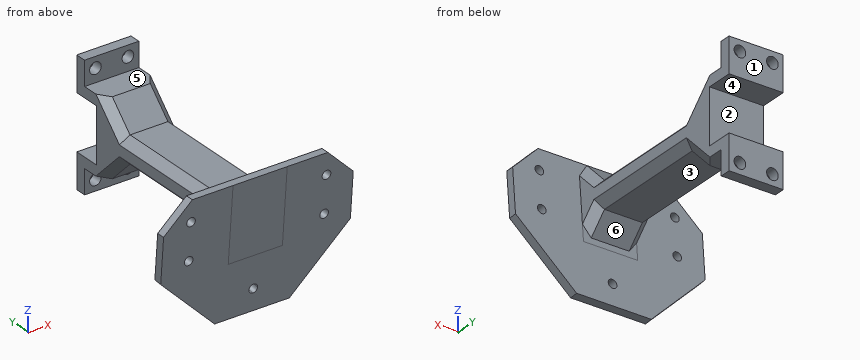
```python
from build123d import *

# Parameters (mm, degrees)
SKETCH1_W           = 20
SKETCH1_H           = 53.344530479
BOSS_EXTRUDE1_DEPTH = 28
BOSS_EXTRUDE2_START = -426.399445517
BOSS_EXTRUDE2_DEPTH = 20
BOSS_EXTRUDE3_DEPTH = 20
SKETCH4_R           = 2.15
CUT_EXTRUDE1_DEPTH  = 10
SKETCH6_R           = 1.6
BOSS_EXTRUDE5_DEPTH = 3
SKETCH7_W           = 104.374043795
SKETCH7_H           = 16.644454458
CUT_EXTRUDE2_DEPTH  = 3
CHAMFER1_SIZE       = 10
CUT_EXTRUDE3_DEPTH  = 60
CHAMFER2_SIZE       = 3


# Read off the part's stored shape, not the designer's step: Boss-Extrude2
with BuildPart() as part:
    # Sketch1 → Boss-Extrude1 (new body)
    with BuildSketch(Plane.XY):
        with Locations((-416.399445517, 267.662547877)):
            Rectangle(SKETCH1_W, SKETCH1_H)
    extrude(amount=-BOSS_EXTRUDE1_DEPTH)

    # Boss-Extrude2 outline → Boss-Extrude2 (add)
    with BuildSketch(Plane.YZ.offset(BOSS_EXTRUDE2_START)):
        Polygon((227.085747643, -28), (240.990282637, -28), (240.990282637, 0), (224.636065064, 0), align=None)
    extrude(amount=BOSS_EXTRUDE2_DEPTH)

    # Sketch3 → Boss-Extrude3 (add)
    with BuildSketch(Plane.ZY.offset(426.399445517)):
        Polygon((-28, 300.334813116), (-37, 300.334813116), (-37, 304.334813116), (-24.1, 304.334813116), (-24.1, 294.334813116), (-28, 294.334813116), align=None)
        Polygon((9, 300.334813116), (9, 304.334813116), (-3.9, 304.334813116), (-3.9, 294.334813116), (0, 294.334813116), (0, 300.334813116), align=None)
    extrude(amount=-BOSS_EXTRUDE3_DEPTH)

    # Sketch4 → Cut-Extrude1 (cut)
    with BuildSketch(Plane(origin=(0, 304.334813116, 0), x_dir=(1, 0, 0), z_dir=(0, 1, 0))):
        with Locations(Location((-422.399445517, 33, 0), (0, 0, 270))):
            Circle(SKETCH4_R)
        with Locations(Location((-410.399445517, 33, 0), (0, 0, 270))):
            Circle(SKETCH4_R)
        with Locations(Location((-410.399445517, -5, 0), (0, 0, 90))):
            Circle(SKETCH4_R)
        with Locations(Location((-422.399445517, -5, 0), (0, 0, 90))):
            Circle(SKETCH4_R)
    extrude(amount=-CUT_EXTRUDE1_DEPTH, mode=Mode.SUBTRACT)

    # Sketch6 → Boss-Extrude5 (add)
    # profile 1 of 2: a face of its own
    with BuildSketch(Plane(origin=(0, 222.929701773, 19.503821668), x_dir=(1, 0, 0), z_dir=(0, -0.9961946980917453, -0.087155742747662))):
        with BuildLine():
            Line((-426.399445517, -19.578323099), (-451.399445517, -19.578323099))
            Line((-451.399445517, -19.578323099), (-451.399445517, -46.472075114))
            Line((-451.399445517, -46.472075114), (-430.186242082, -67.68527855))
            Line((-430.186242082, -67.68527855), (-416.399445517, -67.68527855))
            Line((-416.399445517, -67.68527855), (-416.399445517, -61.28527855))
            ThreePointArc((-416.399445517, -61.28527855), (-417.999445517, -59.68527855), (-416.399445517, -58.08527855))
            Line((-416.399445517, -58.08527855), (-416.399445517, -47.68527855))
            Line((-416.399445517, -47.68527855), (-426.399445517, -47.68527855))
            Line((-426.399445517, -47.68527855), (-426.399445517, -19.578323099))
        make_face()
        with Locations(Location((-441.399445517, -41.472075114, 0), (0, 0, 270))):
            Circle(SKETCH6_R, mode=Mode.SUBTRACT)
        with Locations(Location((-441.399445517, -27.578323099, 0), (0, 0, 270))):
            Circle(SKETCH6_R, mode=Mode.SUBTRACT)
    # profile 2 of 2: a face of its own
    with BuildSketch(Plane(origin=(0, 222.929701773, 19.503821668), x_dir=(1, 0, 0), z_dir=(0, -0.9961946980917453, -0.087155742747662))):
        with BuildLine():
            Line((-416.399445517, -61.28527855), (-416.399445517, -67.68527855))
            Line((-416.399445517, -67.68527855), (-402.612648953, -67.68527855))
            Line((-402.612648953, -67.68527855), (-381.399445517, -46.472075114))
            Line((-381.399445517, -46.472075114), (-381.399445517, -19.578323099))
            Line((-381.399445517, -19.578323099), (-406.399445517, -19.578323099))
            Line((-406.399445517, -19.578323099), (-406.399445517, -47.68527855))
            Line((-406.399445517, -47.68527855), (-416.399445517, -47.68527855))
            Line((-416.399445517, -47.68527855), (-416.399445517, -58.08527855))
            ThreePointArc((-416.399445517, -58.08527855), (-415.268074667, -58.5539077), (-414.799445517, -59.68527855))
            ThreePointArc((-414.799445517, -59.68527855), (-415.268074667, -60.8166494), (-416.399445517, -61.28527855))
        make_face()
        with Locations(Location((-391.399445517, -41.472075114, 0), (0, 0, 270))):
            Circle(SKETCH6_R, mode=Mode.SUBTRACT)
        with Locations(Location((-391.399445517, -27.578323099, 0), (0, 0, 270))):
            Circle(SKETCH6_R, mode=Mode.SUBTRACT)
    extrude(amount=-BOSS_EXTRUDE5_DEPTH)

    # Sketch7 → Cut-Extrude2 (cut)
    with BuildSketch(Plane.XY):
        with Locations((-415.627785026, 222.829224709)):
            Rectangle(SKETCH7_W, SKETCH7_H)
    extrude(amount=CUT_EXTRUDE2_DEPTH, mode=Mode.SUBTRACT)

    # Chamfer1
    chamfer1_edges = [part.edges().sort_by_distance(p)[0] for p in [
        (-451.399445517, 226.141794821, 0),
        (-381.399445517, 226.141794821, 0),
    ]]
    chamfer(chamfer1_edges, length=CHAMFER1_SIZE)

    # Sketch8 → Cut-Extrude3 (cut)
    with BuildSketch(Plane.ZY.offset(426.399445517)):
        Polygon((-28, 290.334813116), (-19, 281.334813116), (-19, 236.647524577), (-25.747394836, 229.90012974), (-28, 230.097207156), align=None)
        Polygon((0, 290.334813116), (-9, 281.334813116), (-9, 236.647524577), (0, 227.647524577), align=None)
    extrude(amount=-CUT_EXTRUDE3_DEPTH, mode=Mode.SUBTRACT)

    # Chamfer2
    chamfer2_edges = [part.edges().sort_by_distance(p)[0] for p in [
        (-406.399445517, 258.991168846, -9),
        (-406.399445517, 258.991168846, -19),
        (-406.399445517, 285.834813116, -23.5),
        (-406.399445517, 233.273827159, -22.373697418),
        (-426.399445517, 233.273827159, -22.373697418),
        (-426.399445517, 258.991168846, -19),
        (-426.399445517, 285.834813116, -23.5),
        (-406.399445517, 285.834813116, -4.5),
        (-406.399445517, 232.147524577, -4.5),
        (-426.399445517, 285.834813116, -4.5),
        (-426.399445517, 258.991168846, -9),
        (-426.399445517, 232.147524577, -4.5),
    ]]
    chamfer(chamfer2_edges, length=CHAMFER2_SIZE)


solid = part.part
```
Verification items for the finished model (mm, model axes). Face numbers are marked on the shaded views. A direction names the side the tool comes from. Coordinates: 2 decimals unless noted, no trailing zeros. Write each loop counter-clockwise with the first axis right and the second up, starting at its lowest first coordinate (ties: lowest second). Pieces come first, ordered by that corner, then holes. Notation, with made-up numbers: (21, -24) - (26, -24) arc R34 cw to (26, 13) - close; hole circle Ø6 at (-27.75, 43). An arc over 180 degrees is marked (long way). One line per question, with ' | ' between items. Start each with the question number.
1. Gauge pin test, flat ends, axial feed: P1, Ø15.5, axis at x = -414, y = 261, coming from the +Z side; P2, Ø3.5, axis at x = -414.5, y = 226.5, coming from the +Z side; P3, Ø10, axis at x = -415.5, z = -32.5, coming from the -Y side; P4, Ø6, axis at y = 236, z = -29.5, coming from the +X side. Record the tip position at first contact, or that the pin passes through.
2. Section check D-D (x = -432.5). Enter the section's corners in (y, z), plus the area to 3 significant figures.
3. Section check B-B (y = 262). Enter the section's corners in (x, z).
4. Access from +Z, -Z, +X, -X, +Y, -Y to the whole of each face (thin tool, end or side, straight path). Record for the marked faces 4, 5 and 6.
5. Section check A-A (z = 5). Enter the section's corners in (x, y).
6. Section check C-C (z = -33). Enter the section's corners in (x, y).
7. Draft check along Z on the marked faces 1, 2 and 3. Enter one of: released by +Z, released by -Z, zero draft, split by the parting line, or undercut.
8. Material ranges on line 1 along X through (y, z) = (301.3, 5); line 2 along Z through (x, y) = (-410.5, 299.5); line 3 along X through (y, z) = (284.5, -11.5), recorded low to high.
Computed values:
1) P1: z = -9 | P2: z = 0 | P3: y = 227.04 | P4: through
2) outline: (224.64, 0) - (228.63, -45.62) - (231.62, -45.36) - (227.65, 0) - close | area: 137 mm²
3) outline: (-426.4, -16) - (-423.4, -19) - (-409.4, -19) - (-406.4, -16) - (-406.4, -12) - (-409.4, -9) - (-423.4, -9) - (-426.4, -12) - close
4) face 4: +X, -X, +Y | face 5: +Z, +X, -X, -Y | face 6: +X, -X
5) outline: (-426.4, 300.33) - (-424.55, 300.33) - (-424.55, 304.33) - (-426.4, 304.33) - close; (-420.25, 300.33) - (-412.55, 300.33) - (-412.55, 304.33) - (-420.25, 304.33) - close; (-408.25, 300.33) - (-406.4, 300.33) - (-406.4, 304.33) - (-408.25, 304.33) - close
6) outline: (-445.17, 227.52) - (-387.63, 227.52) - (-387.89, 230.53) - (-444.9, 230.53) - close; (-426.4, 300.33) - (-424.55, 300.33) - (-424.55, 304.33) - (-426.4, 304.33) - close; (-420.25, 300.33) - (-412.55, 300.33) - (-412.55, 304.33) - (-420.25, 304.33) - close; (-408.25, 300.33) - (-406.4, 300.33) - (-406.4, 304.33) - (-408.25, 304.33) - close
7) face 1: zero draft | face 2: undercut | face 3: released by -Z
8) line 1: -426.4 to -424.55, -420.25 to -412.55, -408.25 to -406.4 | line 2: -28 to -24.1, -3.9 to 0 | line 3: -426.4 to -406.4
